Can you work these out from the model? Positions are in its coordinate system, mm. A direction names the side the tool comes from. Coordinates: 2 decimals unless noted, no trailing zeros. Order: outer loops, then holes, each group sorted by start corner. A loop starts at its lowest first (then second) coordinate and runs counter-clockwise, first axis right, second up. Notation, with made-up numbers: (66, -38) -> (100, -38) arc R18 ccw to (100, -10) -> close; hole circle Ø4 at (-16.75, -7). An arc over 180 degrees is marked (long way). Write item = value, one per line.
```python
from build123d import *

# Parameters (mm, degrees)
ESBO_O1_R                = 12.5
ESBO_O1_R_2              = 5.875
ESBO_O1_R_3              = 1.75
RESSALTO_EXTRUS_O1_DEPTH = 3.8
ESBO_O1_3_R              = 5.875
ESBO_O1_3_R_2            = 4.15
RESSALTO_EXTRUS_O2_DEPTH = 19.5
FILETE1_R                = 0.5


with BuildPart() as part:
    # Esbo_o1 → Ressalto-extrus_o1 (new body)
    with BuildSketch(Plane(origin=(0, 0, 0), x_dir=(1, 0, 0), z_dir=(0, 1, 0))):
        Circle(ESBO_O1_R)
        Circle(ESBO_O1_R_2, mode=Mode.SUBTRACT)
        with Locations((0, 9.25)):
            Circle(ESBO_O1_R_3, mode=Mode.SUBTRACT)
        with Locations((-8.010734985, -4.625)):
            Circle(ESBO_O1_R_3, mode=Mode.SUBTRACT)
        with Locations((8.010734985, -4.625)):
            Circle(ESBO_O1_R_3, mode=Mode.SUBTRACT)
    extrude(amount=RESSALTO_EXTRUS_O1_DEPTH)

    # Esbo_o1_3 → Ressalto-extrus_o2 (add)
    with BuildSketch(Plane(origin=(0, 0, 0), x_dir=(1, 0, 0), z_dir=(0, 1, 0))):
        Circle(ESBO_O1_3_R)
        Circle(ESBO_O1_3_R_2, mode=Mode.SUBTRACT)
    extrude(amount=RESSALTO_EXTRUS_O2_DEPTH)

    # Filete1
    filete1_edges = [part.edges().sort_by_distance(p)[0] for p in [
        (-5.875, 3.8, 0),
    ]]
    fillet(filete1_edges, radius=FILETE1_R)


solid = part.part
```
Item 1: I want a section at D-D, the plane x = -7.75. Please give me the cut outline in (y, z), plus the area to 3 significant figures.
A:
outline = (0, -9.81) -> (3.8, -9.81) -> (3.8, 2.89) -> (0, 2.89) -> close; (0, 6.36) -> (3.8, 6.36) -> (3.8, 9.81) -> (0, 9.81) -> close
area = 61.4 mm2
Item 2: I want a section at C-C, the plane y = 12.25. Please give me the cut outline in (x, z) (3 decimals).
A:
outline = circle Ø11.75 at (0, 0); hole circle Ø8.3 at (0, 0)
Item 3: I want a section at A-A, the plane x = 0. Please give me the cut outline in (y, z) (3 decimals), plus the area to 3 significant figures.
A:
outline = (0, -12.5) -> (3.8, -12.5) -> (3.8, -11) -> (0, -11) -> close; (0, -7.5) -> (3.8, -7.5) -> (3.8, -6.375) arc R0.5 cw to (4.3, -5.875) -> (19.5, -5.875) -> (19.5, -4.15) -> (0, -4.15) -> close; (0, 4.15) -> (19.5, 4.15) -> (19.5, 5.875) -> (4.3, 5.875) arc R0.5 cw to (3.8, 6.375) -> (3.8, 12.5) -> (0, 12.5) -> close
area = 104 mm2
Item 4: For faces 5 (the flat face through (-3, 3.8, -6)), 6 (the flat face through (3, 19.5, 4)), which set-ups out of +Z, -Z, +X, -X, +Y, -Y let a thin tool reach every point of the face, with its end or its side?
A:
face_5 = +Y
face_6 = +Z, -Z, +X, -X, +Y
Item 5: If I drill on probe 1 along Z at (x, y) = (0, 2.55); probe 2 along Z at (x, y) = (0, 6.5) (3 decimals), over which ranges is the centre line in solid material (lowest first)?
A:
probe_1 = -12.5 to -11, -7.5 to -4.15, 4.15 to 12.5
probe_2 = -5.875 to -4.15, 4.15 to 5.875
Item 6: I'm going to push flat-ended pins straight in: P1, Ø4, axis at x = -6.5, z = 7, coming from the +Y side; P2, Ø4, axis at y = 6.5, z = 5, coming from the -X side; P3, Ø1, axis at x = -5, y = 14.5, coming from the +Z side. Where does each tip first touch, or does it pass through?
A:
P1 = 3.8
P2 = -5.05
P3 = 3.78
Item 7: I want a section at B-B, the plane z = 0. Please give me the cut outline in (x, y) (3 decimals), plus the area to 3 significant figures.
A:
outline = (-12.5, 0) -> (-4.15, 0) -> (-4.15, 19.5) -> (-5.875, 19.5) -> (-5.875, 4.3) arc R0.5 cw to (-6.375, 3.8) -> (-12.5, 3.8) -> close; (4.15, 0) -> (12.5, 0) -> (12.5, 3.8) -> (6.375, 3.8) arc R0.5 cw to (5.875, 4.3) -> (5.875, 19.5) -> (4.15, 19.5) -> close
area = 118 mm2
Item 8: If we mould it in two halves opening along Z, with no side actions, what happens to faces 1 (the flat face through (5, 0, 0)), 2 (the cylindrical face through (-6.394, 1.873, 5.295)), 3 (the cylindrical face through (5.604, 11.794, -1.765)), 4 (the cylindrical face through (9.627, 1.873, 5.295))? For each: pulls with the +Z half, pulls with the -Z half, needs draft (parallel to the pull), parting line crosses it, or undercut.
A:
face_1 = needs draft
face_2 = undercut
face_3 = parting line crosses it
face_4 = undercut
